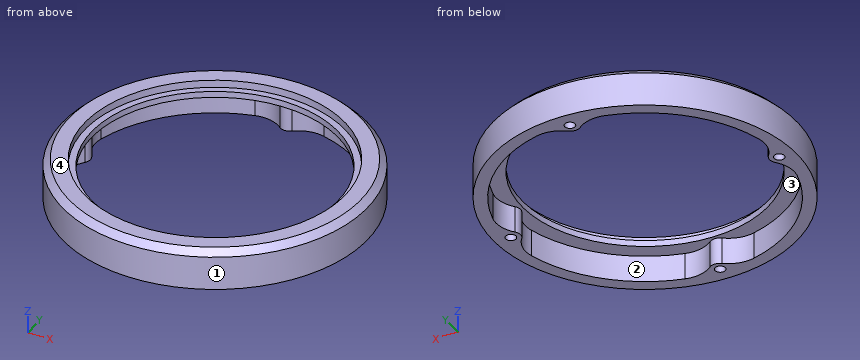
```python
from build123d import *

# Parameters (mm, degrees)
F0_R      = 23.5
F1_DEPTH  = 6.2
F2_T      = -2
F3_SIZE   = 1
F4_R      = 19
F5_DEPTH  = 6.201
F6_R      = 20.05
F7_DEPTH  = 1.15
F8_DEPTH  = 0.1
F9_R      = 1.5
F10_DEPTH = 4.1
F11_R     = 5
F12_R     = 0.8
F13_DEPTH = 4.8


with BuildPart() as f1:
    # F0 (on Top) → F1 (new body)
    with BuildSketch(Plane.XY):
        Circle(F0_R)
    extrude(amount=F1_DEPTH)

    # F2
    f2_openings = [f1.faces().sort_by_distance(p)[0] for p in [
        (0, 0, 0),
    ]]
    offset(amount=F2_T, openings=f2_openings)

    # F3
    f3_edges = [f1.edges().sort_by_distance(p)[0] for p in [
        (-23.5, 0, 6.2),
    ]]
    chamfer(f3_edges, length=F3_SIZE)

    # F4 (on face) → F5 (cut, through all)
    with BuildSketch(Plane.XY.offset(6.2)):
        Circle(F4_R)
    extrude(amount=-F5_DEPTH, mode=Mode.SUBTRACT)

    # F6 (on face) → F7 (cut)
    with BuildSketch(Plane.XY.offset(6.2)):
        Circle(F6_R)
    extrude(amount=-F7_DEPTH, mode=Mode.SUBTRACT)

    # F8 (add): a face of the model
    f8_faces = [f1.faces().sort_by_distance(p)[0] for p in [
        (-20.8918881682, 0, 4.2),
    ]]
    extrude(f8_faces, amount=F8_DEPTH)

    # F9 (on face) → F10 (join, through all)
    with BuildSketch(Plane(origin=(0, 0, 4.1), x_dir=(1, 0, 0), z_dir=(0, 0, -1))):
        with Locations((0, 21)):
            Circle(F9_R)
        with Locations((-21, 0)):
            Circle(F9_R)
        with Locations((0, -21)):
            Circle(F9_R)
        with Locations((21, 0)):
            Circle(F9_R)
    extrude(amount=F10_DEPTH)

    # F11
    f11_edges = [f1.edges().sort_by_distance(p)[0] for p in [
        (21.452381, -1.430158, 2.05),
        (21.452381, 1.430158, 2.05),
        (-1.430158, -21.452381, 2.05),
        (1.430158, -21.452381, 2.05),
        (-21.452381, 1.430158, 2.05),
        (-21.452381, -1.430158, 2.05),
        (-1.430158, 21.452381, 2.05),
        (1.430158, 21.452381, 2.05),
    ]]
    fillet(f11_edges, radius=F11_R)

    # F12 (on face) → F13 (cut)
    with BuildSketch(Plane(origin=(0, 0, 0), x_dir=(1, 0, 0), z_dir=(0, 0, -1))):
        with Locations((0, -21)):
            Circle(F12_R)
        with Locations((21, 0)):
            Circle(F12_R)
        with Locations((0, 21)):
            Circle(F12_R)
        with Locations((-21, 0)):
            Circle(F12_R)
    extrude(amount=-F13_DEPTH, mode=Mode.SUBTRACT)


solid = f1.part
```
Geometry: final body of the model. Coordinates: model frame, mm. Face numbers are marked on the shaded views. Coordinates: 2 decimals unless noted, no trailing zeros. Write each loop counter-clockwise with the first axis right and the second up, starting at its lowest first coordinate (ties: lowest second). Pieces come first, ordered by that corner, then holes. Notation, with made-up numbers: M 36,81.25 L 93,81.25 A19 cw 93,91.25 Z; hole C 13,-11 d5. An arc over 180 degrees is marked long. Answer as CSV lines item,"result". Start each with the question number.
Q1. Mould query, pull axis X, two halves, no side actions, for the marked faces 1, 2, 3 and 4. Classes: released by +X, released by -X, zero draft, split by the parting line, or undercut.
Q2. Pin query (flat end, axial travel): P1, Ø24, axis at x = 0, y = 0, coming from the +Z side; P2, Ø1.5, axis at x = -12.5, z = 1, coming from the -Y side; P3, Ø0.5, axis at x = 0, y = -21, coming from the -Z side; P4, Ø3, axis at y = -14.5, z = 2.5, coming from the +X side. Return the tip coordinate at first contact, or that it passes through.
Q3. Cut plane C-C on z = 3.5. Count the separate pieces of the cut face and the enclosed holes in it, then the cut area to 3 significant figures.
Q4. Line query: line 1 (Y direction, x = 0, z = 4.6); line 2 (Y direction, x = 0, z = 1.9); line 3 (Z direction, x = 17.5, y = -12). Output: solid intervals per line, ascending. Write a range as from..to.
Q5. Cut plane A-A on x = 0. Return the cut outline in (y, z).
Findings below:
1,face 1,"split by the parting line"
1,face 2,"undercut"
1,face 3,"undercut"
1,face 4,"zero draft"
2,P1,"passes through"
2,P2,"stops at y = -20.35"
2,P3,"stops at z = 4.8"
2,P4,"stops at x = 19.58"
3,separate pieces,"1"
3,enclosed holes,"5"
3,area,"308 mm2"
4,line 1,"y = -23.5..-21.8, -20.2..-19, 19..20.2, 21.8..23.5"
4,line 2,"y = -23.5..-21.8, -20.2..-19.5, 19.5..20.2, 21.8..23.5"
4,line 3,"z = 4.1..6.2"
5,outline,"M -23.5,0 L -21.8,0 L -21.8,4.8 L -20.2,4.8 L -20.2,0 L -19.5,0 L -19.5,4.1 L -19,4.1 L -19,5.05 L -20.05,5.05 L -20.05,6.2 L -22.5,6.2 L -23.5,5.2 Z; M 19,4.1 L 19.5,4.1 L 19.5,0 L 20.2,0 L 20.2,4.8 L 21.8,4.8 L 21.8,0 L 23.5,0 L 23.5,5.2 L 22.5,6.2 L 20.05,6.2 L 20.05,5.05 L 19,5.05 Z"
